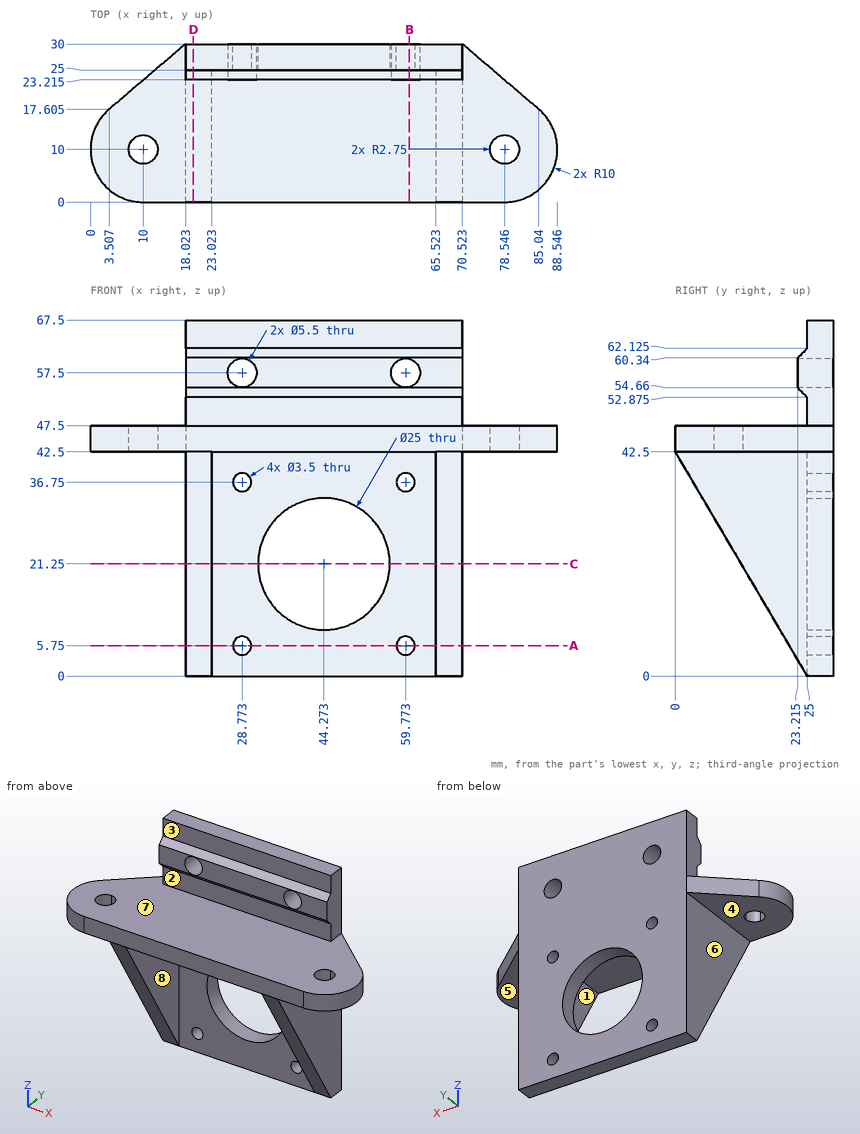
Answer from the drawing. Dimensions are ordinates in mm from the lowest x, y and z of the part. A direction names the side the tool comes from. Coordinates: 2 decimals unless noted, no trailing zeros. Loops run counter-clockwise (first coordinate to the right, second up) from the corner with the lowest first, then second, coordinate; pieces in that order, holes last. Notation, with made-up numbers: (54, 80.5) - (78, 80.5) arc R33 ccw to (78, 119.5) - close; hole circle Ø10 at (39.5, -13.5). An arc over 180 degrees is marked (long way). Use a Markdown table: item, result.
Item 1: Find section B-B, the plane x = 60.5. State how many separate pieces and enclosed holes the cut face has, and give its area (3 significant figures).
Evaluation:
| item | result |
|---|---|
| separate pieces | 4 |
| enclosed holes | 0 |
| area | 408 mm2 |
Item 2: Find section D-D, the plane x = 19.5. Determine the outline of the cut face in (y, z) (1 decimal).
Evaluation:
| item | result |
|---|---|
| outline | (0, 42.5) - (25, 0) - (30, 0) - (30, 67.5) - (25, 67.5) - (25, 62.1) - (23.2, 60.3) - (23.2, 54.7) - (25, 52.9) - (25, 47.5) - (0, 47.5) - close |
Item 3: Find section A-A, the plane z = 5.75. Determine the outline of the cut face in (x, y), and give its area (3 significant figures).
Evaluation:
| item | result |
|---|---|
| outline | (18.02, 21.62) - (23.02, 21.62) - (23.02, 25) - (27.02, 25) - (27.02, 30) - (18.02, 30) - close; (30.52, 25) - (58.02, 25) - (58.02, 30) - (30.52, 30) - close; (61.52, 25) - (65.52, 25) - (65.52, 21.62) - (70.52, 21.62) - (70.52, 30) - (61.52, 30) - close |
| area | 261 mm2 |
Item 4: Consider probe 1 along X at (y, z) = (11.75, 24); probe 2 along Z at (x, y) = (30, 24.5) (1 decimal); probe 3 along Z at (x, y) = (80.5, 4.75). Determine where each line is inside the solid, lowest interval first. Write a range as from..to.
Evaluation:
| item | result |
|---|---|
| probe 1 | x = 18.02..23.02, 65.52..70.52 |
| probe 2 | z = 42.5..47.5, 53.4..55, 60..61.6 |
| probe 3 | z = 42.5..47.5 |
Item 5: Given pin 1 Ø1.5 at (y, z) = (16.5, 29.5) entering from -X; pin 2 Ø3 at (y, z) = (22.5, 54.5) entering from +X; pin 3 Ø4.5 at (x, z) = (45.5, 50) entering from -Y; pin 4 Ø5.5 at (x, z) = (28.77, 36.75) entering from +Y, each flat-ended and moving along its own axis, determine where each tip first touches the part or whether it passes through.
Evaluation:
| item | result |
|---|---|
| pin 1 | stops at x = 18.02 |
| pin 2 | stops at x = 70.52 |
| pin 3 | stops at y = 25 |
| pin 4 | stops at y = 30 |
Item 6: The mould has two halves that part along X. Classify the marked faces 6, 7 and 8: +X half, -X half, draft (parallel to the pull), parting line (faces both ways), or undercut.
Evaluation:
| item | result |
|---|---|
| face 6 | -X half |
| face 7 | draft |
| face 8 | undercut |
Item 7: For the marked faces 1, 2, 3, 4 and 5, determine the directions among +Z, -Z, +X, -X, +Y, -Y from which every point of the face is accessible in a straight line to the end or side of a thin tool.
Evaluation:
| item | result |
|---|---|
| face 1 | -Z, -Y |
| face 2 | +X, -X, -Y |
| face 3 | +Z, +X, -X, -Y |
| face 4 | -Z, -X, +Y, -Y |
| face 5 | -Z, +X, +Y, -Y |
Item 8: Find section C-C, the plane z = 21.25. Determine the outline of the cut face in (x, y).
Evaluation:
| item | result |
|---|---|
| outline | (18.02, 12.5) - (23.02, 12.5) - (23.02, 25) - (31.77, 25) - (31.77, 30) - (18.02, 30) - close; (56.77, 25) - (65.52, 25) - (65.52, 12.5) - (70.52, 12.5) - (70.52, 30) - (56.77, 30) - close |
